Autodesk Inventor part; units mm, degrees
ref_plane "Work Plane1" through (-14, 0, 0) normal (1, 0, 0) x (0, 1, 0)
ref_plane "XZ Plane" through (0, 0, 0) normal (0, 1, 0) x (-1, 0, 0)
ref_plane "XY Plane" through (0, 0, 0) normal (0, 0, 1) x (1, 0, 0)
sketch "Sketch1" plane through (0, 0, 0) normal (0, 1, 0) x (-1, 0, 0)
  circle A0 centre (0, 0) radius 20
  line L0 (0, 20) -> (20, 20)
  line L1 (20, 20) -> (20, -20)
  line L2 (20, -20) -> (0, -20)
  line L3 (0, -20) -> (0, 20)
  dimension "d0" = 40
extrude "Extrusion1" add sketch "Sketch1" along normal blind 15
sketch "Sketch2" plane through (0, 15, 0) normal (0, 1, 0) x (1, 0, 0)
  circle A0 centre (0, 0) radius 15.25
  dimension "d3" = 30.5
extrude "Extrusion2" cut sketch "Sketch2" against normal up to next
sketch "Sketch3" plane through (0, 15, 0) normal (0, 1, 0) x (1, 0, 0)
  line L0 (10, -11) -> (30, -11)
  line L1 (30, -11) -> (30, 11)
  line L2 (30, 11) -> (10, 11)
  line L3 (10, 11) -> (10, -11)
  arc A0 (0, -20) -> (0, 20) centre (0, 0) ccw
  line L4 (10, -11) -> (30, 11) construction
  line L5 (30, -11) -> (10, 11) construction
  point P0 (20, 0)
  dimension "d6" = 22
  dimension "d7" = 20
extrude "Extrusion3" cut sketch "Sketch3" against normal up to next
ref_plane "Work Plane1" through (-14, 0, 0) normal (1, 0, 0) x (0, 1, 0)
sketch "Sketch7" plane through (-14, 0, 0) normal (1, 0, 0) x (0, 1, 0)
  circle A0 centre (7.5, 0) radius 4.25
  line L0 (0, -15.25) -> (0, 15.25)
  point P0 (0, 0)
  point P1 (0, -11)
  point P2 (0, 11)
  dimension "d18" = 8.5
  dimension "d19" = 7.5
extrude "Extrusion4" cut sketch "Sketch7" against normal blind 3
sketch "Sketch8" plane through (-17, 7.5, 0) normal (1, 0, 0) x (0, 0, -1)
  circle A0 centre (0, 0) radius 2.375
  point P0 (0, -7.5)
  dimension "d22" = 4.75
extrude "Extrusion5" cut sketch "Sketch8" against normal up to next
properties part number "60mL_falcon_holder"
Can you work these out from the model? Positions are in its coordinate system, mm. A direction names the side the tool comes from. Round coordinates to 2 decimals unless told otherwise and drop trailing zeros. Write each loop counter-clockwise with the first axis right and the second up, starting at its lowest first coordinate (ties: lowest second). Pieces come first, ordered by that corner, then holes. Notation, with made-up numbers: M 36,68 L 78,68 A19 cw 78,79 Z; hole C 37.5,41 d2. An arc over 180 degrees is marked long. Use CSV: the item, a comma, the result in double quotes.
(1) Imagine slicing it at C-C (y = 13.5). Write out the boundary of the cut face in (x, z), plus the area to 3 significant figures.
Check values:
outline,"M -20,-20 L 0,-20 A20 ccw 16.7,-11 L 10.56,-11 A15.25 cw long 10.56,11 L 16.7,11 A20 ccw 0,20 L -20,20 Z"
area,"585 mm^2"
(2) I'm going to push flat-ended pins straight in: pin 1 (1.8 mm diameter, centred on x = 12.5, y = 10, fed in from -Z); pin 2 (7 mm diameter, centred on x = 12, y = 10, fed in from +Z). Where does each tip first touch, or does it pass through?
Check values:
pin 1,"z = -16.29"
pin 2,"z = 18.1"
(3) We'd pull the mould along Y, two halves only. Please class faces 1 (the flat face through (-17, 9.3, -1.8)), 2 (the flat face through (-18, 15, 0)), 3 (the flat face through (14, 8, 11)): +Y half, -Y half, draft (parallel to the pull), parting line (faces both ways), or undercut.
Check values:
face 1,"undercut"
face 2,"+Y half"
face 3,"draft"
(4) Imagine slicing it at B-B (z = 12.5). Write out the boundary of the cut face in (x, y), plus the area to 3 significant figures.
Check values:
outline,"M -20,0 L -8.74,0 L -8.74,15 L -20,15 Z; M 8.74,0 L 15.61,0 L 15.61,15 L 8.74,15 Z"
area,"272 mm^2"
(5) Imagine slicing it at D-D (x = -10). Write out the boundary of the cut face in (y, z), plus the area to 3 significant figures.
Check values:
outline,"M 0,-20 L 15,-20 L 15,-11.51 L 0,-11.51 Z; M 0,11.51 L 15,11.51 L 15,20 L 0,20 Z"
area,"255 mm^2"
(6) On a 3-axis mill with a long thin cutter (end or side, diameter ignored), from which of +Z, -Z, +X, -X, +Y, -Y can I reach the whole of each face in a straight line? I mean faces 4 (the cylindrical face through (-18.479, 9.855, 0.309)), 5 (the cylindrical face through (-16.068, 4.368, 2.872)), 6 (the flat face through (14, 8, -11)). Say none if no direction works.
Check values:
face 4,"+X, -X"
face 5,"+X"
face 6,"+X, +Y, -Y"
(7) Imagine slicing it at A-A (y = 6.5). Write out the boundary of the cut face in (x, z), plus the area to 3 significant figures.
Check values:
outline,"M -20,-20 L 0,-20 A20 ccw 16.7,-11 L 10.56,-11 A15.25 cw -14.68,-4.13 L -17,-4.13 L -17,-2.15 L -20,-2.15 Z; M -20,2.15 L -17,2.15 L -17,4.13 L -14.68,4.13 A15.25 cw 10.56,11 L 16.7,11 A20 ccw 0,20 L -20,20 Z"
area,"556 mm^2"
(8) I need wall thicknesses on line 1 along Y through (x, z) = (-18, 0) (3 decimals); line 2 along Y through (x, z) = (-16.45, 0); line 3 along Z through (x, y) = (-15.4, 7.5). Which ranges of each line are inside material? Lowest first, please.
Check values:
line 1,"0 to 5.125, 9.875 to 15"
line 2,"0 to 3.25, 11.75 to 15"
line 3,"-20 to -4.25, 4.25 to 20"
